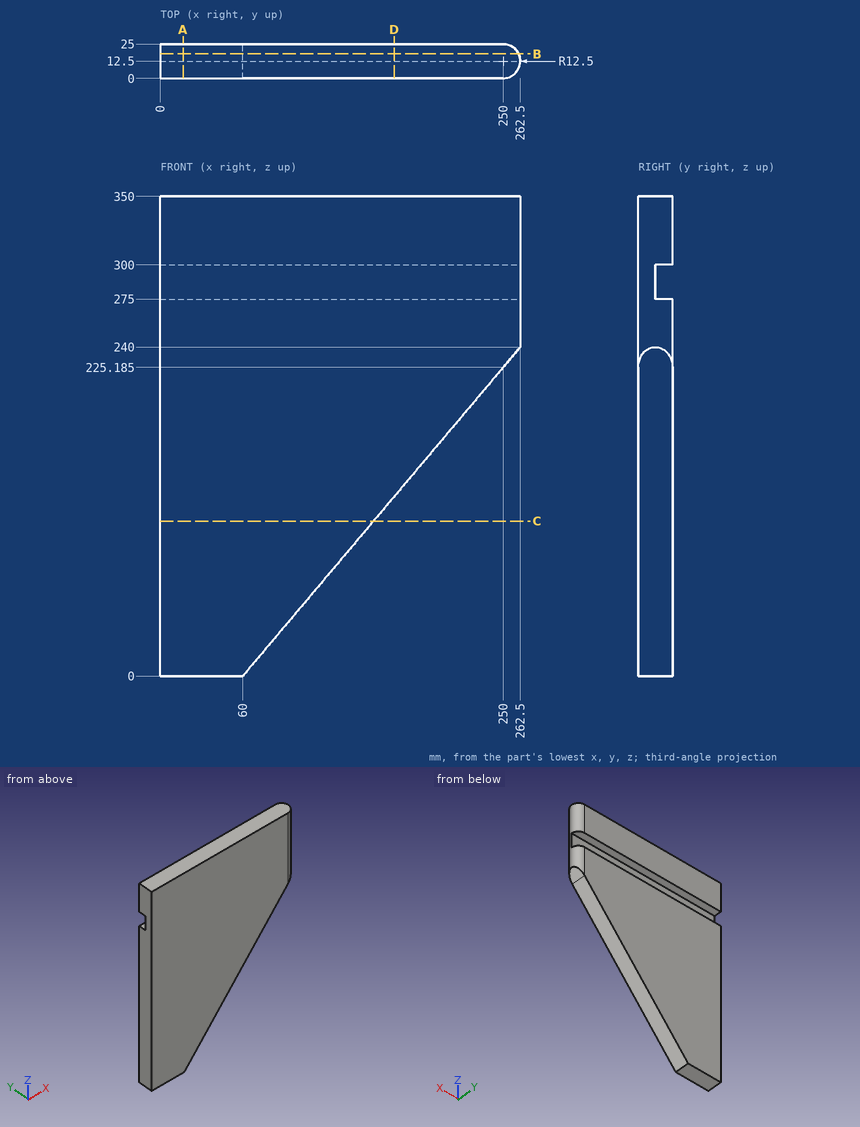
Verification items for this drawing (mm, ordinates from the low corner). Coordinates: 2 decimals unless noted, no trailing zeros. Order: outer loops, then holes, each group sorted by start corner. A loop starts at its lowest first (then second) coordinate and runs counter-clockwise, first axis right, second up. Notation, with made-up numbers: M 1.25,4 L 12.25,4 A25 ccw 12.25,19 Z; hole C 16,21.25 d11. An arc over 180 degrees is marked long. Use CSV: the item, a comma, the result in double quotes.
Item 1: Cross-section at A-A on x = 16.5. Record the cut outline in (y, z).
Returned:
outline,"M 0,0 L 25,0 L 25,275 L 12.5,275 L 12.5,300 L 25,300 L 25,350 L 0,350 Z"
Item 2: Cross-section at D-D on x = 170.5. Record the cut outline in (y, z), then the cut area to 3 significant figures.
Returned:
outline,"M 0,130.96 L 25,130.96 L 25,275 L 12.5,275 L 12.5,300 L 25,300 L 25,350 L 0,350 Z"
area,"5,160 mm2"
Item 3: Cross-section at B-B on y = 17.75. Record the cut outline in (x, z) (1 decimal).
Returned:
outline,"M 0,0 L 60,0 L 261.3,238.6 L 261.3,275 L 0,275 Z; M 0,300 L 261.3,300 L 261.3,350 L 0,350 Z"
Item 4: Cross-section at C-C on z = 113. Record the cut outline in (x, y).
Returned:
outline,"M 0,0 L 155.34,0 L 155.34,25 L 0,25 Z"
Item 5: Gauge pin test, flat ends, axial feed: pin 1 Ø4 at (x, y) = (176.5, 19) entering from -Z; pin 2 Ø3 at (y, z) = (13, 144.5) entering from +X; pin 3 Ø12.5 at (x, z) = (169, 292.5) entering from +Y. Record the tip position at first contact, or that the pin passes through.
Returned:
pin 1,"stops at z = 135.7"
pin 2,"stops at x = 183.19"
pin 3,"stops at y = 12.5"
Item 6: Thickness scan on line 1 along Z through (x, y) = (14.5, 18); line 2 along Z through (x, y) = (124, 13.25); line 3 along X through (y, z) = (13, 304.5). Record the ranges inside material, lowest first.
Returned:
line 1,"z = 0 to 275, 300 to 350"
line 2,"z = 75.85 to 275, 300 to 350"
line 3,"x = 0 to 262.49"
